```python
from build123d import *

# Parameters (mm, degrees)
F0_R     = 1.5
F1_DEPTH = 2
F2_R     = 2.5
F3_DEPTH = 5
F5_DEPTH = 25


with BuildPart() as f1:
    # F0 (on Front) → F1 (new body)
    with BuildSketch(Plane.XZ):
        with BuildLine():
            ThreePointArc((22.7870577302, -9), (24.0679549857, -4.5807797158), (24.5, 0))
            ThreePointArc((24.5, 0), (-4.5807797158, 24.0679549857), (-22.7870577302, -9))
            Line((-22.7870577302, -9), (0, -9))
            Line((0, -9), (22.7870577302, -9))
        make_face()
        with Locations((-12.5, 0)):
            Circle(F0_R, mode=Mode.SUBTRACT)
        with BuildLine():
            ThreePointArc((1, 0), (0.7071067812, -0.7071067812), (0, -1))
            ThreePointArc((0, -1), (-0.7071067812, 0.7071067812), (1, 0))
        make_face(mode=Mode.SUBTRACT)
        with Locations((12.5, 0)):
            Circle(F0_R, mode=Mode.SUBTRACT)
    extrude(amount=F1_DEPTH)

    # F2 (on face) → F3 (join)
    with BuildSketch(Plane.XZ.offset(2)):
        with Locations((0, 16)):
            Circle(F2_R)
    extrude(amount=F3_DEPTH)

    # F4 (on face) → F5 (cut)
    with BuildSketch(Plane.XZ.offset(2)):
        with BuildLine():
            ThreePointArc((24.5, 0), (0, 24.5), (-24.5, 0))
            add(Edge.make_bspline(
                [(-24.5, 0), (-16.3333333333, 9.25), (-8.1666666667, 18.5), (0, 18.5)],
                knots=[0, 0, 0, 0, 0.5, 0.5, 0.5, 0.5], degree=3))
            add(Edge.make_bspline(
                [(0, 18.5), (8.1666666667, 18.5), (16.3333333333, 9.25), (24.5, 0)],
                knots=[0.5, 0.5, 0.5, 0.5, 1, 1, 1, 1], degree=3))
        make_face()
    extrude(amount=-F5_DEPTH, mode=Mode.SUBTRACT)


solid = f1.part
```
CAD build for the part. Positions are in the model's coordinates, mm. Give positions to 0.01 mm unless a question says otherwise; leave off trailing zeros. Loops run counter-clockwise (first coordinate to the right, second up) from the corner with the lowest first, then second, coordinate; pieces in that order, holes last. Notation, with made-up numbers: M -20.5,45 L 29.5,45 A21 cw 29.5,82 Z; hole C 83.25,-9.5 d11. An arc over 180 degrees is marked long. Use one line per item in the form item = value.
Item 1: Slice it at A-A (y = -2.75). List the corners of the cut face in (x, z).
Determined:
outline = C 0,16 d5
Item 2: Two-plate mould, pull along Z, no slides. Class faces 1 (the face through (11, -1, 0)), 2 (the face through (-0.54, -4.46, 13.56)), 3 (the face through (0, -2, 2)): pulls with the +Z half, pulls with the -Z half, needs draft (parallel to the pull), parting line crosses it, or undercut.
Determined:
face_1 = undercut
face_2 = parting line crosses it
face_3 = needs draft
Item 3: Slice it at B-B (z = -3). List the corners of the cut face in (x, y).
Determined:
outline = M -24.32,-2 L 24.32,-2 L 24.32,0 L -24.32,0 Z
Item 4: Flat gauge pins, fed straight in: pin 1 (2 mm diameter, centred on x = -1.5, y = -5, fed in from -Z); pin 2 (1.6 mm diameter, centred on x = 0, z = 0, fed in from -Y); pin 3 (10 mm diameter, centred on x = -10.5, z = 5, fed in from -Y). Where does each tip first touch, or does it go through?
Determined:
pin_1 = 13.55
pin_2 = through
pin_3 = -2
Item 5: Drill centre lines: probe 1 along Z at (x, y) = (0, -1.35); probe 2 along Y at (x, z) = (20.5, -6.75); probe 3 along Z at (x, y) = (-6, -1.5). Where is each one in solid material? Low to high. Write a range as from..to.
Determined:
probe_1 = -9..-1, 1..18.5
probe_2 = -2..0
probe_3 = -9..16.97
